Check sheet for the drawn part. Datum: minimum x, y, z corner. Units: mm. Coordinates: 2 decimals unless noted, no trailing zeros. Order: outer loops, then holes, each group sorted by start corner. A loop starts at its lowest first (then second) coordinate and runs counter-clockwise, first axis right, second up.
Q1. Thickness scan on line 1 (Z direction, x = 2.5, y = 5.25); line 2 (X direction, y = 2.75, z = 3); line 3 (Z direction, x = 3, y = 3.25). Record the ranges inside material, lowest first.
Q2. Cross-section at C-C, the plane y = 3. Record the boundary of the cut face in (x, z), and give its area (3 significant figures).
Q3. Cross-section at D-D, the plane y = 6.75. Record the boundary of the cut face in (x, z), and give its area (3 significant figures).
Q4. Cross-section at B-B, the plane z = 3. Record the boundary of the cut face in (x, y), and give its area (3 significant figures).
Q5. Cross-section at A-A, the plane x = 3.5. Record the boundary of the cut face in (y, z).
Q6. Depth check by flat-ended pin: P1, Ø1.9, axis at x = 3.5, z = 21, coming from the +Y side. Enter the tip coordinate at first touch or a pass-through.
Q7. Draft check along Z on the marked faces 1, 2 and 3. Enter one of: pulls with the +Z half, pulls with the -Z half, needs draft (parallel to the pull), parting line crosses it, or undercut.
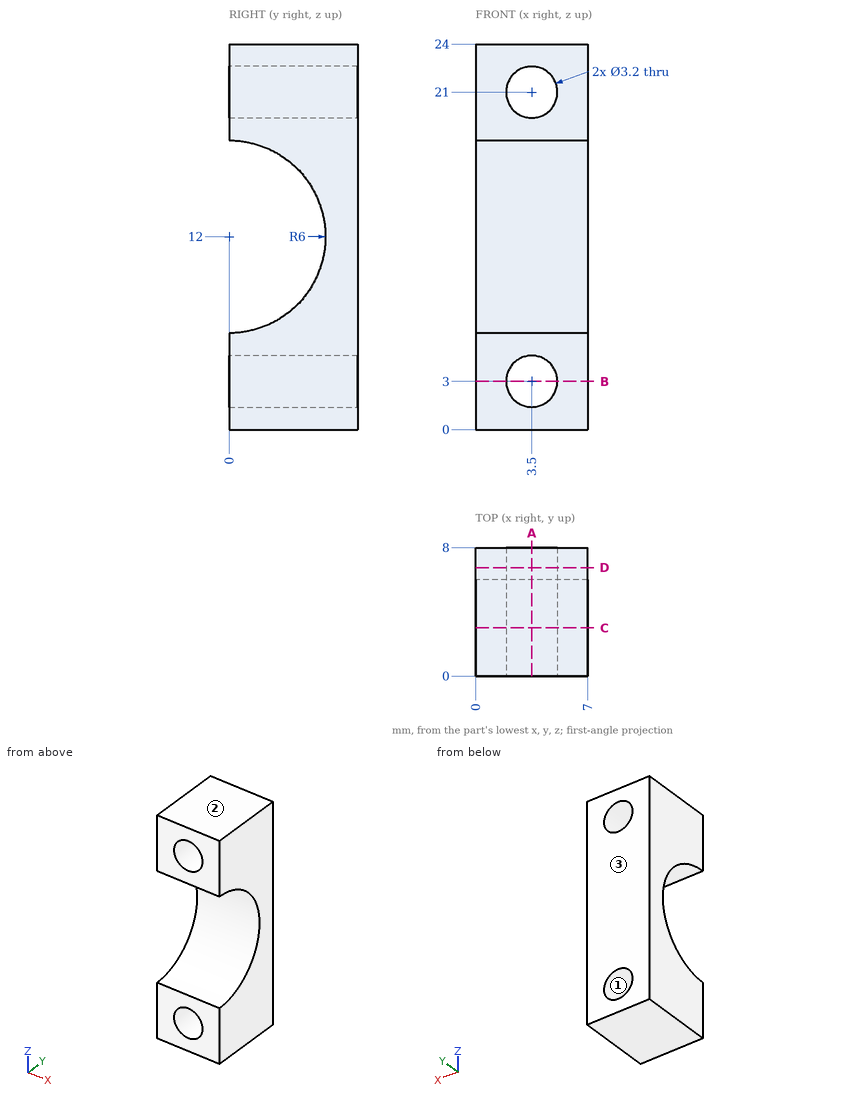
Check values:
1. line 1: z = 0 to 1.75, 4.25 to 9.1, 14.9 to 19.75, 22.25 to 24
1. line 2: x = 0 to 1.9, 5.1 to 7
1. line 3: z = 0 to 1.48, 4.52 to 6.96, 17.04 to 19.48, 22.52 to 24
2. outline: (0, 0) - (7, 0) - (7, 6.8) - (0, 6.8) - close; (0, 17.2) - (7, 17.2) - (7, 24) - (0, 24) - close; hole circle Ø3.2 at (3.5, 3); hole circle Ø3.2 at (3.5, 21)
2. area: 79.2 mm2
3. outline: (0, 0) - (7, 0) - (7, 24) - (0, 24) - close; hole circle Ø3.2 at (3.5, 3); hole circle Ø3.2 at (3.5, 21)
3. area: 152 mm2
4. outline: (0, 0) - (1.9, 0) - (1.9, 8) - (0, 8) - close; (5.1, 0) - (7, 0) - (7, 8) - (5.1, 8) - close
4. area: 30.4 mm2
5. outline: (0, 0) - (8, 0) - (8, 1.4) - (0, 1.4) - close; (0, 4.6) - (8, 4.6) - (8, 19.4) - (0, 19.4) - (0, 18) arc R6 cw to (0, 6) - close; (0, 22.6) - (8, 22.6) - (8, 24) - (0, 24) - close
6. P1: passes through
7. face 1: undercut
7. face 2: pulls with the +Z half
7. face 3: needs draft
